from build123d import *

# Parameters (mm, degrees)
BOSS_EXTRUDE1_DEPTH = 5
SKETCH2_R           = 21.5
CUT_EXTRUDE1_DEPTH  = 74.068461049
SKETCH3_R           = 3.15
CUT_EXTRUDE2_DEPTH  = 74.068461049
SKETCH12_R          = 2.9
CUT_EXTRUDE3_DEPTH  = 3
SKETCH13_R          = 1.75
CUT_EXTRUDE4_DEPTH  = 73.958892535
CUT_EXTRUDE5_DEPTH  = 3
CUT_EXTRUDE6_DEPTH  = 1.5


with BuildPart() as part:
    # Sketch1 → Boss-Extrude1 (new body)
    with BuildSketch(Plane.XY):
        with BuildLine():
            Line((25, 65), (-25, 65))
            ThreePointArc((-25, 65), (-30.656854249, 62.656854249), (-33, 57))
            Line((-33, 57), (-33, -57))
            ThreePointArc((-33, -57), (-30.656854249, -62.656854249), (-25, -65))
            Line((-25, -65), (25, -65))
            ThreePointArc((25, -65), (30.656854249, -62.656854249), (33, -57))
            Line((33, -57), (33, 57))
            ThreePointArc((33, 57), (30.656854249, 62.656854249), (25, 65))
        make_face()
    extrude(amount=BOSS_EXTRUDE1_DEPTH)

    # Sketch2 → Cut-Extrude1 (cut, through all)
    with BuildSketch(Plane.XY.offset(5)):
        Circle(SKETCH2_R)
    extrude(amount=-CUT_EXTRUDE1_DEPTH, mode=Mode.SUBTRACT)

    # Sketch3 → Cut-Extrude2 (cut, through all)
    with BuildSketch(Plane.XY.offset(5)):
        with Locations((0, 26.5)):
            Circle(SKETCH3_R)
        with Locations((0, -26.5)):
            Circle(SKETCH3_R)
    extrude(amount=-CUT_EXTRUDE2_DEPTH, mode=Mode.SUBTRACT)

    # Sketch12 → Cut-Extrude3 (cut)
    with BuildSketch(Plane.XY.offset(5)):
        with Locations((-27.75, 59.75)):
            Circle(SKETCH12_R)
        with Locations(Location((27.75, 59.75, 0), (0, 0, 180))):
            Circle(SKETCH12_R)
        with Locations(Location((-27.75, -59.75, 0), (0, 0, 180))):
            Circle(SKETCH12_R)
        with Locations((27.75, -59.75)):
            Circle(SKETCH12_R)
    extrude(amount=-CUT_EXTRUDE3_DEPTH, mode=Mode.SUBTRACT)

    # Sketch13 → Cut-Extrude4 (cut, through all)
    with BuildSketch(Plane.XY.offset(2)):
        with Locations((-27.75, 59.75)):
            Circle(SKETCH13_R)
        with Locations(Location((27.75, 59.75, 0), (0, 0, 180))):
            Circle(SKETCH13_R)
        with Locations((27.75, -59.75)):
            Circle(SKETCH13_R)
        with Locations(Location((-27.75, -59.75, 0), (0, 0, 180))):
            Circle(SKETCH13_R)
    extrude(amount=-CUT_EXTRUDE4_DEPTH, mode=Mode.SUBTRACT)

    # Sketch14 → Cut-Extrude5 (cut)
    with BuildSketch(Plane.XY.offset(5)):
        with BuildLine():
            Line((-5.5, 26.5), (-5.5, -26.5))
            ThreePointArc((-5.5, -26.5), (0, -32), (5.5, -26.5))
            Line((5.5, -26.5), (5.5, 26.5))
            ThreePointArc((5.5, 26.5), (0, 32), (-5.5, 26.5))
        make_face()
    extrude(amount=-CUT_EXTRUDE5_DEPTH, mode=Mode.SUBTRACT)

    # Sketch15 → Cut-Extrude6 (cut)
    with BuildSketch(Plane.XY.offset(5)):
        with BuildLine():
            Line((-2.5, 65), (-2.5, 31.398979486))
            ThreePointArc((-2.5, 31.398979486), (0, 32), (2.5, 31.398979486))
            Line((2.5, 31.398979486), (2.5, 65))
            Line((2.5, 65), (-2.5, 65))
        make_face()
        with BuildLine():
            Line((-27.75, 13.75), (-20.879116361, 13.75))
            ThreePointArc((-20.879116361, 13.75), (-14.747047157, 20.187238547), (-6.75, 24.071508054))
            Line((-6.75, 24.071508054), (-6.75, 59.75))
            Line((-6.75, 59.75), (-21.75, 59.75))
            ThreePointArc((-21.75, 59.75), (-23.507359313, 55.507359313), (-27.75, 53.75))
            Line((-27.75, 53.75), (-27.75, 13.75))
        make_face()
        with BuildLine():
            Line((27.75, 13.75), (20.879116361, 13.75))
            ThreePointArc((20.879116361, 13.75), (14.747047157, 20.187238547), (6.75, 24.071508054))
            Line((6.75, 24.071508054), (6.75, 59.75))
            Line((6.75, 59.75), (21.75, 59.75))
            ThreePointArc((21.75, 59.75), (23.507359313, 55.507359313), (27.75, 53.75))
            Line((27.75, 53.75), (27.75, 13.75))
        make_face()
        with BuildLine():
            Line((27.75, -53.75), (27.75, -13.75))
            Line((27.75, -13.75), (20.879116361, -13.75))
            ThreePointArc((20.879116361, -13.75), (14.747047157, -20.187238547), (6.75, -24.071508054))
            Line((6.75, -24.071508054), (6.75, -59.75))
            Line((6.75, -59.75), (21.75, -59.75))
            ThreePointArc((21.75, -59.75), (23.507359313, -55.507359313), (27.75, -53.75))
        make_face()
        with BuildLine():
            Line((2.5, -65), (2.5, -31.398979486))
            ThreePointArc((2.5, -31.398979486), (0, -32), (-2.5, -31.398979486))
            Line((-2.5, -31.398979486), (-2.5, -65))
            Line((-2.5, -65), (2.5, -65))
        make_face()
        with BuildLine():
            Line((-6.75, -59.75), (-6.75, -24.071508054))
            ThreePointArc((-6.75, -24.071508054), (-14.747047157, -20.187238547), (-20.879116361, -13.75))
            Line((-20.879116361, -13.75), (-27.75, -13.75))
            Line((-27.75, -13.75), (-27.75, -53.75))
            ThreePointArc((-27.75, -53.75), (-23.507359313, -55.507359313), (-21.75, -59.75))
            Line((-21.75, -59.75), (-6.75, -59.75))
        make_face()
    extrude(amount=-CUT_EXTRUDE6_DEPTH, mode=Mode.SUBTRACT)


solid = part.part
Input: part model. Units: mm. Frame: model coordinates. A direction names the side the tool comes from. Give positions to 0.01 mm unless a question says otherwise; leave off trailing zeros. Write each loop counter-clockwise with the first axis right and the second up, starting at its lowest first coordinate (ties: lowest second). Pieces come first, ordered by that corner, then holes. Notation, with made-up numbers: M -35.5,-23 L -0.5,-23 A22 cw -0.5,9 Z; hole C 75,12 d9. An arc over 180 degrees is marked long. Use one line per item in the form item = value.
1. Mould query, pull axis Y, two halves, no side actions, for faces 1 (the face through (5.5, -24, 4)), 2 (the face through (0, 65, 2)), 3 (the face through (-22, 1, 0)), 4 (the face through (-30, -60, 2)). Classes: released by +Y, released by -Y, zero draft, split by the parting line, or undercut.
Outcome:
face_1 = undercut
face_2 = released by +Y
face_3 = zero draft
face_4 = undercut
2. Cut plane A-A on y = 0. Return loops of the section in (x, z), and give its area (3 significant figures).
Outcome:
outline = M -33,0 L -21.5,0 L -21.5,5 L -33,5 Z; M 21.5,0 L 33,0 L 33,5 L 21.5,5 Z
area = 115 mm²
3. Ray query, L1, parallel to Y at x = 0, z = 1.25; L2, parallel to X at y = 36.5, z = 3.65; L3, parallel to Y at x = -4.5, z = 4.55. Return the intervals inside material, ascending.
Outcome:
L1 = -65 to -29.65, -23.35 to -21.5, 21.5 to 23.35, 29.65 to 65
L2 = -33 to -27.75, -6.75 to -2.5, 2.5 to 6.75, 27.75 to 33
L3 = -65 to -29.66, 29.66 to 65
4. Cut plane B-B on x = 0. Return loops of the section in (y, z).
Outcome:
outline = M -65,0 L -29.65,0 L -29.65,2 L -32,2 L -32,3.5 L -65,3.5 Z; M -23.35,0 L -21.5,0 L -21.5,2 L -23.35,2 Z; M 21.5,0 L 23.35,0 L 23.35,2 L 21.5,2 Z; M 29.65,0 L 65,0 L 65,3.5 L 32,3.5 L 32,2 L 29.65,2 Z
5. Reachability of faces 5 (the face through (30.719, 62.594, 2.465)), 6 (the face through (-28.38, 56.92, 3.52)), 7 (the face through (0, -48, 3.5)) from +Z, -Z, +X, -X, +Y, -Y: full face, straight path, thin tool, end or side. Return the list, or none.
Outcome:
face_5 = +Z, -Z, +X, +Y
face_6 = +Z
face_7 = +Z, +Y, -Y
6. Cut plane C-C on z = 0.75. Return loops of the section in (x, y).
Outcome:
outline = M -33,-57 A8 ccw -25,-65 L 25,-65 A8 ccw 33,-57 L 33,57 A8 ccw 25,65 L -25,65 A8 ccw -33,57 Z; hole C -27.75,-59.75 d3.5; hole C -27.75,59.75 d3.5; hole C 0,0 d43; hole C 0,-26.5 d6.3; hole C 0,26.5 d6.3; hole C 27.75,-59.75 d3.5; hole C 27.75,59.75 d3.5
7. Cut plane D-D on y = -45. Return loops of the section in (x, z).
Outcome:
outline = M -33,0 L 33,0 L 33,5 L 27.75,5 L 27.75,3.5 L 6.75,3.5 L 6.75,5 L 2.5,5 L 2.5,3.5 L -2.5,3.5 L -2.5,5 L -6.75,5 L -6.75,3.5 L -27.75,3.5 L -27.75,5 L -33,5 Z
8. First-contact query: P1, Ø23, axis at x = 13.5, y = -39.5, coming from the +Z side; P2, Ø3.5, axis at x = -0.5, y = 28, coming from the +Z side; P3, Ø10.5, axis at x = 17, y = 40.5, coming from the +Z side. Flat tips, straight axial feed; report the tip coordinate or a pass-through.
Outcome:
P1 = 5
P2 = 2
P3 = 3.5
